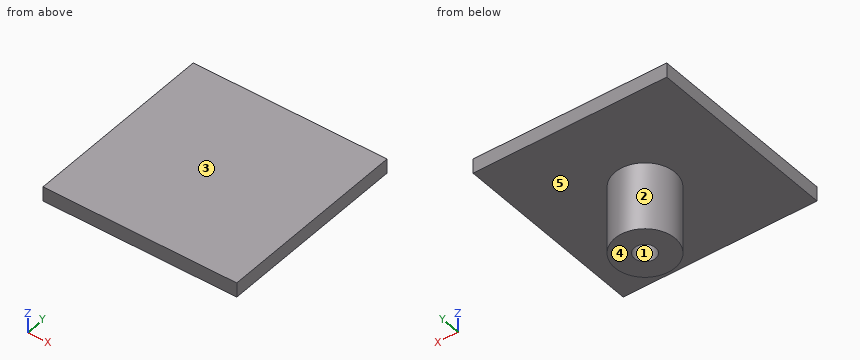
from build123d import *

# Parameters (mm, degrees)
SKETCH_2_W        = 20
SKETCH_2_H        = 20
EXTRUDE_348_DEPTH = 1.5
SKETCH_3_R        = 3.1
SKETCH_3_R_2      = 1.1
EXTRUDE_476_DEPTH = 7


with BuildPart() as part:
    # Эскиз2 → Extrude 348 (new body)
    with BuildSketch(Plane.XY):
        Rectangle(SKETCH_2_W, SKETCH_2_H)
    extrude(amount=EXTRUDE_348_DEPTH)

    # Эскиз3 → Extrude 476 (add)
    with BuildSketch(Plane.XY):
        Circle(SKETCH_3_R)
        Circle(SKETCH_3_R_2, mode=Mode.SUBTRACT)
    extrude(amount=-EXTRUDE_476_DEPTH)


solid = part.part
The listing builds one solid part. Answer for the finished solid, in the listing's coordinates (mm). Face numbers are marked on the shaded views. A direction names the side the tool comes from. Round coordinates to 2 decimals unless told otherwise and drop trailing zeros. Order: outer loops, then holes, each group sorted by start corner. A loop starts at its lowest first (then second) coordinate and runs counter-clockwise, first axis right, second up. Notation, with made-up numbers: (-37, 50.25) -> (-3, 50.25) arc R31 cw to (-3, 74.25) -> close; hole circle Ø9 at (-38, 80.25). An arc over 180 degrees is marked (long way). Write each question's results on one line, items separated by ' | '. Start each with the question number.
Q1. Which of the six approach directions +Z, -Z, +X, -X, +Y, -Y give full straight-line access (tool end or side, diameter ignored) to the marked faces 4 and 5?
Q2. Straight lines are drawn through the part: probe 1 along Y at (x, z) = (0, -1.75); probe 2 along Z at (x, y) = (-7, -5.5); probe 3 along X at (y, z) = (1, -3). For each, find the intervals that lie inside material, in ascending order. Write a range as from..to.
Q3. The mould has two halves that part along Y. Classify the marked faces 1, 2 and 3: pulls with the +Y half, pulls with the -Y half, needs draft (parallel to the pull), parting line crosses it, or undercut.
Q4. Find section D-D (x = 2.75). Determine the outline of the cut face in (y, z).
Q5. Find section C-C (z = -1). Determine the outline of the cut face in (x, y).
Q6. Find section A-A (x = 0). Determine the outline of the cut face in (y, z), then the cut area to 3 significant figures.
Q7. This flat-tipped pin is pushed along its axis until it touches: pin 1 (2 mm diameter, centred on x = 0, y = 0, fed in from -Z). Where does it stop, or does it pass through?
Worked answers:
1) face 4: -Z, +X, -X, +Y, -Y | face 5: -Z
2) probe 1: y = -3.1..-1.1, 1.1..3.1 | probe 2: z = 0..1.5 | probe 3: x = -2.93..-0.46, 0.46..2.93
3) face 1: undercut | face 2: parting line crosses it | face 3: needs draft
4) outline: (-10, 0) -> (-1.43, 0) -> (-1.43, -7) -> (1.43, -7) -> (1.43, 0) -> (10, 0) -> (10, 1.5) -> (-10, 1.5) -> close
5) outline: circle Ø6.2 at (0, 0); hole circle Ø2.2 at (0, 0)
6) outline: (-10, 0) -> (-3.1, 0) -> (-3.1, -7) -> (-1.1, -7) -> (-1.1, 0) -> (1.1, 0) -> (1.1, -7) -> (3.1, -7) -> (3.1, 0) -> (10, 0) -> (10, 1.5) -> (-10, 1.5) -> close | area: 58.0 mm2
7) pin 1: stops at z = 0
